from build123d import *

# Parameters (mm, degrees)
SKETCH1_R               = 2.4892
BOSS_EXTRUDE1_DEPTH     = 6.35
BOSS_EXTRUDE2_START     = -6.35
BOSS_EXTRUDE2_DEPTH     = 19.05
BOSS_EXTRUDE2_START_2   = -6.555460136
BOSS_EXTRUDE2_2_DEPTH   = 19.460920272
BOSS_EXTRUDE2_START_3   = -10
BOSS_EXTRUDE2_3_DEPTH   = 3.65
CUT_EXTRUDE1_DEPTH      = 27.910448217
CUT_EXTRUDE1_DEPTH_BACK = 27.910448217
SKETCH3_W               = 2.179354936
SKETCH3_H               = 6.35
CUT_EXTRUDE2_DEPTH      = 31.98795935
CUT_EXTRUDE2_DEPTH_BACK = 31.98795935


with BuildPart() as part:
    # Sketch1 → Boss-Extrude1 (new body)
    with BuildSketch(Plane(origin=(0, 0, 0), x_dir=(1, 0, 0), z_dir=(0, 1, 0))):
        with BuildLine():
            Line((9.525, -17.889269346), (-0.578271622, -16.817120786))
            Line((-0.578271622, -16.817120786), (-6.35, 0))
            Line((-6.35, 0), (12.7, 0))
            Line((12.7, 0), (12.7, -6.35))
            ThreePointArc((12.7, -6.35), (15.186560179, -13.240601753), (9.525, -17.889269346))
        make_face()
        with Locations(Location((9.525, -11.43, 0), (0, 0, 270))):
            Circle(SKETCH1_R, mode=Mode.SUBTRACT)
    extrude(amount=BOSS_EXTRUDE1_DEPTH)

    # Boss-Extrude2: read off the stored shape, not the designer's step
    # Boss-Extrude2 outline → Boss-Extrude2 (add)
    with BuildSketch(Plane.YZ.offset(BOSS_EXTRUDE2_START)):
        with BuildLine():
            ThreePointArc((11.551615481, -6.35), (12.905510296, -4.996105185), (11.551615481, -3.642210371))
            Line((11.551615481, -3.642210371), (6.35, 0))
            Line((6.35, 0), (0, 0))
            Line((0, 0), (-5.201615481, -3.642210371))
            ThreePointArc((-5.201615481, -3.642210371), (-6.555510296, -4.996105185), (-5.201615481, -6.35))
            Line((-5.201615481, -6.35), (11.551615481, -6.35))
        make_face()
    extrude(amount=BOSS_EXTRUDE2_DEPTH)

    # Boss-Extrude2 2 outline → Boss-Extrude2 2 (add)
    with BuildSketch(Plane(origin=(0, 0, 0), x_dir=(1, 0, 0), z_dir=(0, 1, 0)).offset(BOSS_EXTRUDE2_START_2)):
        Polygon((-8.529354936, 6.35), (-6.35, 0), (-6.35, 6.35), align=None)
    extrude(amount=BOSS_EXTRUDE2_2_DEPTH)

    # Boss-Extrude2 3 outline → Boss-Extrude2 3 (cut)
    with BuildSketch(Plane.YZ.offset(BOSS_EXTRUDE2_START_3)):
        with BuildLine():
            Line((12.905460136, 0), (6.35, 0))
            Line((6.35, 0), (11.551615481, -3.642210371))
            ThreePointArc((11.551615481, -3.642210371), (12.504834401, -4.034645431), (12.905460136, -4.984450993))
            Line((12.905460136, -4.984450993), (12.905460136, 0))
        make_face()
        with BuildLine():
            ThreePointArc((12.905460136, -5.007759378), (12.504834401, -5.95756494), (11.551615481, -6.35))
            Line((11.551615481, -6.35), (12.905460136, -6.35))
            Line((12.905460136, -6.35), (12.905460136, -5.007759378))
        make_face()
        with BuildLine():
            Line((0, 0), (-6.555460136, 0))
            Line((-6.555460136, 0), (-6.555460136, -4.984450993))
            ThreePointArc((-6.555460136, -4.984450993), (-6.154834401, -4.034645431), (-5.201615481, -3.642210371))
            Line((-5.201615481, -3.642210371), (0, 0))
        make_face()
        with BuildLine():
            ThreePointArc((-5.201615481, -6.35), (-6.154834401, -5.95756494), (-6.555460136, -5.007759378))
            Line((-6.555460136, -5.007759378), (-6.555460136, -6.35))
            Line((-6.555460136, -6.35), (-5.201615481, -6.35))
        make_face()
    extrude(amount=BOSS_EXTRUDE2_3_DEPTH, mode=Mode.SUBTRACT)

    # Sketch3 → Cut-Extrude1 (cut, two sides: drawn at the far end of the back side and taken through both)
    with BuildSketch(Plane.XZ.offset(-CUT_EXTRUDE1_DEPTH_BACK)):
        with Locations((-7.439677468, -3.175)):
            Rectangle(SKETCH3_W, SKETCH3_H)
    extrude(amount=CUT_EXTRUDE1_DEPTH + CUT_EXTRUDE1_DEPTH_BACK, mode=Mode.SUBTRACT)

    # Sketch4 → Cut-Extrude2 (cut, two sides: drawn at the far end of the back side and taken through both)
    with BuildSketch(Plane.ZY.offset(6.35).offset(-CUT_EXTRUDE2_DEPTH_BACK)):
        with BuildLine():
            ThreePointArc((-5.842, -5.006022622), (-4.983704134, -5.864318488), (-4.125408268, -5.006022622))
            Line((-4.125408268, -5.006022622), (-0.620153491, 0))
            Line((-0.620153491, 0), (0, 0))
            Line((0, 0), (-3.642210371, -5.201615481))
            ThreePointArc((-3.642210371, -5.201615481), (-4.996105185, -6.555510296), (-6.35, -5.201615481))
            Line((-6.35, -5.201615481), (-6.35, 11.551615481))
            ThreePointArc((-6.35, 11.551615481), (-4.996105185, 12.905510296), (-3.642210371, 11.551615481))
            Line((-3.642210371, 11.551615481), (0, 6.35))
            Line((0, 6.35), (-0.620153491, 6.35))
            Line((-0.620153491, 6.35), (-4.125408268, 11.356022622))
            ThreePointArc((-4.125408268, 11.356022622), (-4.983704134, 12.214318488), (-5.842, 11.356022622))
            Line((-5.842, 11.356022622), (-5.842, -5.006022622))
        make_face()
    extrude(amount=CUT_EXTRUDE2_DEPTH + CUT_EXTRUDE2_DEPTH_BACK, mode=Mode.SUBTRACT)


solid = part.part
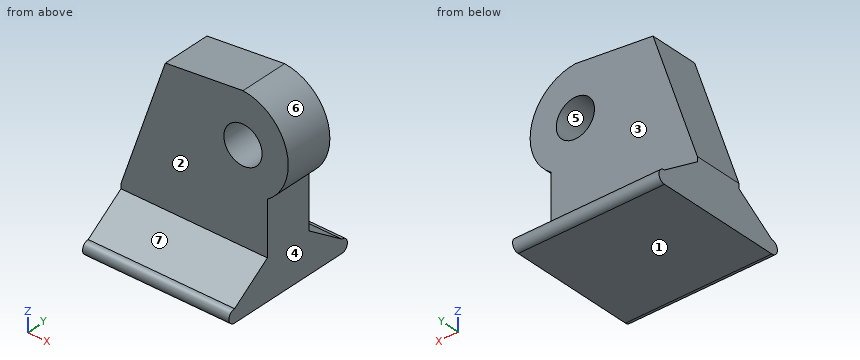
For this review, take the finished solid that the model builds, in its own axes (mm). Face numbers are marked on the shaded views. A direction names the side the tool comes from. Give positions to 0.01 mm unless a question says otherwise; leave off trailing zeros. Loops run counter-clockwise (first coordinate to the right, second up) from the corner with the lowest first, then second, coordinate; pieces in that order, holes last.
Item 1: Take a section at A-A, the plane x = 9. State the section outline as (y, z) points, and give its area (3 significant figures).
Item 2: Insertion check: pin 1 (3 mm diameter, centred on x = -1.5, z = 0.5, fed in from +Y); pin 2 (12 mm diameter, centred on x = -2, z = 12, fed in from -Y); pin 3 (6 mm diameter, centred on y = 3, z = 1, fed in from +X). Each pin has a flat end and moves straight along its axis. Give the tip position at first contact, or say it passes through.
Item 3: For line 1 along Y through (x, z) = (-4.5, 3.5); line 2 along X through (y, z) = (4.5, 11.5), list the stretches that pass through material, from the lowest coordinate up.
Item 4: Tool access review of the marked faces 1, 2 and 3: name each direction out of +Z, -Z, +X, -X, +Y, -Y from which nothing blocks a thin tool from reaching the whole face with its end or side.
Item 5: Take a section at B-B, the plane y = 4.75. State the section outline as (x, z) points (3 decimals), and give its area (3 significant figures).
Item 6: Take a section at D-D, the plane x = -3.25. State the section outline as (y, z) points.
Item 7: Take a section at C-C, the plane z = 11.43. State the section outline as (x, y) points, and give its area (3 significant figures).
Item 8: Draft analysis for pull direction Z (two halves, no side actions). For the marked faces 4, 5, 6 and 7, state which applies: +Z half, -Z half, draft (parallel to the pull), parting line (faces both ways), or undercut.
Calculated:
1. outline: (-5.01, -5.84) - (11.36, -5.84) arc R0.86 ccw to (11.36, -4.13) - (6.35, -0.62) - (6.35, 9) - (0, 9) - (0, -0.62) - (-5.01, -4.13) arc R0.86 ccw to start; (0, 13.86) - (6.35, 13.86) - (6.35, 17.83) - (0, 17.83) - close
1. area: 156 mm2
2. pin 1: stops at y = 6.89
2. pin 2: stops at y = 0
2. pin 3: stops at x = 12.7
3. line 1: y = 0 to 6.35
3. line 2: x = -2.4 to 7.04, 12.01 to 15.41
4. face 1: -Z, +X, -X, +Y, -Y
4. face 2: +Z, +X, -X, -Y
4. face 3: +Z, +X, -X, +Y
5. outline: (-6.35, -5.842) - (12.7, -5.842) - (12.7, 6.35) arc R6.35 ccw to (9.525, 17.889) - (-0.578, 16.817) - (-6.35, 0) - close; hole circle Ø4.978 at (9.525, 11.43)
5. area: 391 mm2
6. outline: (-5.01, -5.84) - (11.36, -5.84) arc R0.86 ccw to (11.36, -4.13) - (6.35, -0.62) - (6.35, 9.03) - (0, 9.03) - (0, -0.62) - (-5.01, -4.13) arc R0.86 ccw to start
7. outline: (-2.43, 0) - (7.04, 0) - (7.04, 6.35) - (-2.43, 6.35) - close; (12.01, 0) - (15.41, 0) - (15.41, 6.35) - (12.01, 6.35) - close
7. area: 81.7 mm2
8. face 4: draft
8. face 5: undercut
8. face 6: parting line
8. face 7: +Z half
